Build history of the part. All positions in model axes, mm. Round coordinates to 2 decimals unless told otherwise and drop trailing zeros. Write each loop counter-clockwise with the first axis right and the second up, starting at its lowest first coordinate (ties: lowest second). Pieces come first, ordered by that corner, then holes.
Item 1: Band-saw the part on C-C, the plane z = 35. Write the cut outline in (x, y), then the cut area to 3 significant figures.
Item 2: Drop flat-ended pins along their axis: pin 1 Ø13 at (y, z) = (0, 35) entering from +X; pin 2 Ø1.5 at (x, z) = (1, -1) entering from +Y; pin 3 Ø4 at (x, z) = (-3, 9.5) entering from +Y; pin 4 Ø1 at (x, y) = (1.5, -7) entering from +Z. Give the stop position or say it passes through.
Item 3: Band-saw the part on B-B, the plane x = -1. Write the cut outline in (y, z).
Item 4: Wall check: probe 1 along Z at (x, y) = (-2.75, -3.5); probe 2 along Y at (x, z) = (1.25, 35); probe 3 along Z at (x, y) = (0.5, 12). Give the ranges that are in metal, low to high.
Item 5: Band-saw the part on D-D, the plane z = 8. Write the cut outline in (x, y).
Item 6: Band-saw the part on A-A, the plane y = 0. Write the cut outline in (x, z).
Item 7: Mould opens along Z. For faces 1 (the cylindrical face through (-0.1, -2.4, 38.2)), 2 (the flat face through (-0.06, -14.18, -25.44)), 3 (the flat face through (-0.06, 14.18, 25.44)) say: +Z half, -Z half, draft (parallel to the pull), parting line (faces both ways), or undercut.
```python
from build123d import *

# Parameters (mm, degrees)
BOSS_EXTRUDE1_DEPTH      = 4
BOSS_EXTRUDE1_DEPTH_BACK = 4
SKETCH1_R                = 4


with BuildPart() as part:
    # Sketch1 → Boss-Extrude1 (new, two sides: drawn at the far end of the back side and taken through both)
    with BuildSketch(Plane(origin=(0, 0, 0), x_dir=(0, 0, -1), z_dir=(1, 0, 0)).offset(-BOSS_EXTRUDE1_DEPTH_BACK)):
        with BuildLine():
            ThreePointArc((-38.75, 6.495190528), (-42.5, 0), (-38.75, -6.495190528))
            Line((-38.75, -6.495190528), (-12.5, -21.650635095))
            ThreePointArc((-12.5, -21.650635095), (0, -25), (12.5, -21.650635095))
            Line((12.5, -21.650635095), (38.75, -6.495190528))
            ThreePointArc((38.75, -6.495190528), (42.5, 0), (38.75, 6.495190528))
            Line((38.75, 6.495190528), (12.5, 21.650635095))
            ThreePointArc((12.5, 21.650635095), (0, 25), (-12.5, 21.650635095))
            Line((-12.5, 21.650635095), (-38.75, 6.495190528))
        make_face()
        with Locations((-35, 0)):
            Circle(SKETCH1_R, mode=Mode.SUBTRACT)
        with Locations((35, 0)):
            Circle(SKETCH1_R, mode=Mode.SUBTRACT)
    extrude(amount=BOSS_EXTRUDE1_DEPTH + BOSS_EXTRUDE1_DEPTH_BACK)


solid = part.part
```
Results:
1. outline: (-4, -8.66) - (4, -8.66) - (4, -4) - (-4, -4) - close; (-4, 4) - (4, 4) - (4, 8.66) - (-4, 8.66) - close
1. area: 74.6 mm2
2. pin 1: stops at x = 4
2. pin 2: stops at y = 25
2. pin 3: stops at y = 23.85
2. pin 4: stops at z = 38.74
3. outline: (-21.65, -12.5) - (-6.5, -38.75) arc R7.5 ccw to (6.5, -38.75) - (21.65, -12.5) arc R25 ccw to (21.65, 12.5) - (6.5, 38.75) arc R7.5 ccw to (-6.5, 38.75) - (-21.65, 12.5) arc R25 ccw to start; hole circle Ø8 at (0, -35); hole circle Ø8 at (0, 35)
4. probe 1: z = -41.63 to -36.94, -33.06 to 33.06, 36.94 to 41.63
4. probe 2: y = -8.66 to -4, 4 to 8.66
4. probe 3: z = -29.22 to 29.22
5. outline: (-4, -23.69) - (4, -23.69) - (4, 23.69) - (-4, 23.69) - close
6. outline: (-4, -42.5) - (4, -42.5) - (4, -39) - (-4, -39) - close; (-4, -31) - (4, -31) - (4, 31) - (-4, 31) - close; (-4, 39) - (4, 39) - (4, 42.5) - (-4, 42.5) - close
7. face 1: undercut
7. face 2: -Z half
7. face 3: +Z half
